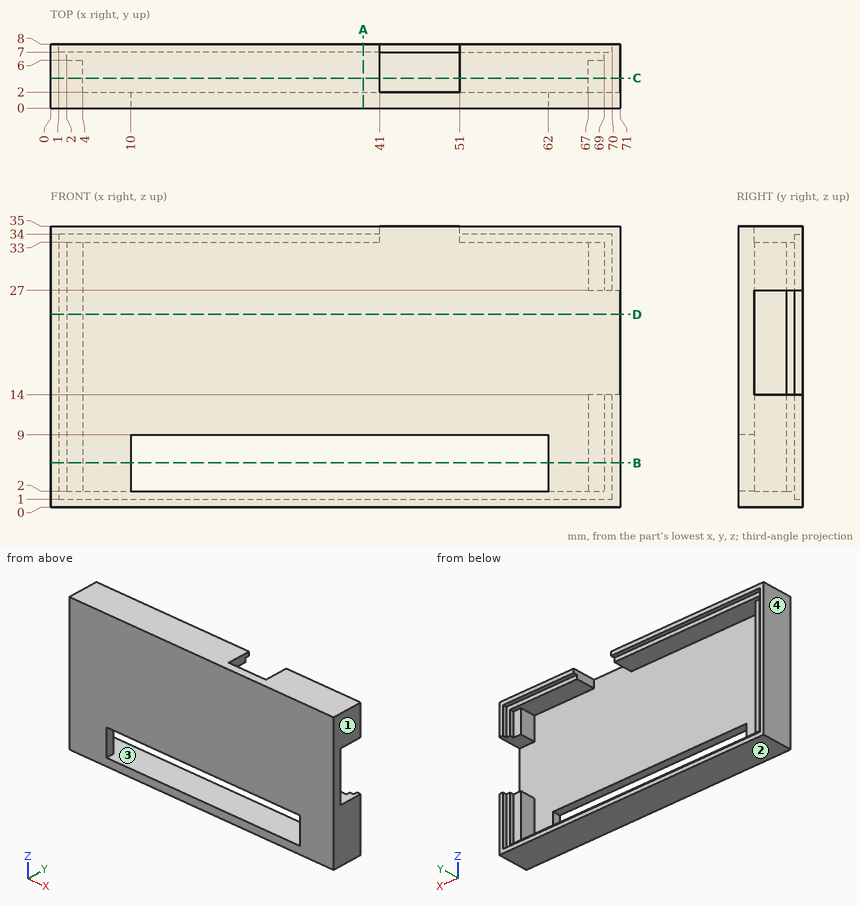
Verification items for this drawing (mm, ordinates from the low corner). Coordinates: 2 decimals unless noted, no trailing zeros. Write each loop counter-clockwise with the first axis right and the second up, starting at its lowest first coordinate (ties: lowest second). Pieces come first, ordered by that corner, then holes. Notation, with made-up numbers: M 31.5,-15 L 88.5,-15 A20 cw 88.5,12 Z; hole C 86,-22.5 d3. An arc over 180 degrees is marked long. One line per item, written item: value. Start each with the question number.
(1) Sectioned sample at D-D, the plane z = 24. Enter the section's corners in (x, y).
(2) Sectioned sample at B-B, the plane z = 5.5. Enter the section's corners in (x, y), and give its area (3 significant figures).
(3) Release check for a two-part mould opening along X. For the marked faces 1, 2, 3 and 4 record: released by +X, released by -X, zero draft, split by the parting line, or undercut.
(4) Depth check by flat-ended pin: pin 1 (1 mm diameter, centred on x = 3, z = 20, fed in from +Y); pin 2 (2 mm diameter, centred on x = 68.5, z = 30.5, fed in from +Y). Enter the tip coordinate at first touch or a pass-through.
(5) Sectioned sample at C-C, the plane y = 3.75. Enter the section's corners in (x, z), and give its area (3 significant figures).
(6) Scan lines: line 1 along Z through (x, y) = (38.5, 3.5); line 2 along X through (y, z) = (4, 6.5); line 3 along Z through (x, y) = (8, 7.25). Record each from-to range of solid material in increasing order. Write a range as [from, to].
(7) Sectioned sample at A-A, the plane x = 39. Enter the section's corners in (y, z), and give its area (3 significant figures).
Filled sheet:
1. outline: M 0,0 L 71,0 L 71,2 L 4,2 L 4,6 L 2,6 L 2,7 L 1,7 L 1,8 L 0,8 Z
2. outline: M 0,0 L 10,0 L 10,2 L 4,2 L 4,6 L 2,6 L 2,7 L 1,7 L 1,8 L 0,8 Z; M 62,0 L 71,0 L 71,8 L 70,8 L 70,7 L 69,7 L 69,6 L 67,6 L 67,2 L 62,2 Z
2. area: 76.0 mm²
3. face 1: released by +X
3. face 2: zero draft
3. face 3: undercut
3. face 4: released by -X
4. pin 1: y = 6
4. pin 2: y = 7
5. outline: M 0,0 L 71,0 L 71,14 L 67,14 L 67,2 L 4,2 L 4,33 L 41,33 L 41,35 L 0,35 Z; M 51,33 L 67,33 L 67,27 L 71,27 L 71,35 L 51,35 Z
5. area: 460 mm²
6. line 1: [0, 2], [33, 35]
6. line 2: [0, 4], [67, 71]
6. line 3: [0, 1], [34, 35]
7. outline: M 0,0 L 8,0 L 8,1 L 7,1 L 7,2 L 0,2 Z; M 0,9 L 2,9 L 2,33 L 7,33 L 7,34 L 8,34 L 8,35 L 0,35 Z
7. area: 78.0 mm²
